The listing builds one solid part. Answer for the finished solid, in the listing's coordinates (mm). Face numbers are marked on the shaded views. Round coordinates to 2 decimals unless told otherwise and drop trailing zeros. Loops run counter-clockwise (first coordinate to the right, second up) from the corner with the lowest first, then second, coordinate; pieces in that order, holes last. Notation, with made-up numbers: (-15.5, -36.5) - (6.5, -36.5) arc R23 ccw to (6.5, -5.5) - close; hole circle Ø8 at (-39.75, 3). An arc over 180 degrees is marked (long way). Write item = value, one per line. Start each with the question number.
1) Section B-B, the plane x = 519 is taken. Determine the outline of the cut face in (y, z).
2) Section C-C, the plane y = 316.5 is taken. Determine the outline of the cut face in (x, z), and give its area (3 significant figures).
3) For a pull along Z with two mould halves and no side action, classify the marked faces 1 and 2 as released by +Z, released by -Z, zero draft, split by the parting line, or undercut.
4) Section A-A, the plane z = 0.45 is taken. Give the number of separate pieces and of enclosed holes in the cut face, and give its area (3 significant figures).
5) Given pin 1 Ø1.3 at (x, z) = (446.5, 1.5) entering from +Y; pin 2 Ø1 at (y, z) = (461.5, 1.5) entering from -X; pin 3 Ø0.5 at (x, z) = (446, 2) entering from -Y, each flat-ended and moving along its own axis, determine where each tip first touches the part or whether it passes through.
6) Straight lines are drawn through the part: line 1 along Y through (x, z) = (457, 2.9); line 2 along Y through (x, z) = (452.5, 0.1); line 3 along X through (y, z) = (567, 2.35). For each, find the intervals that lie inside material, in ascending order.
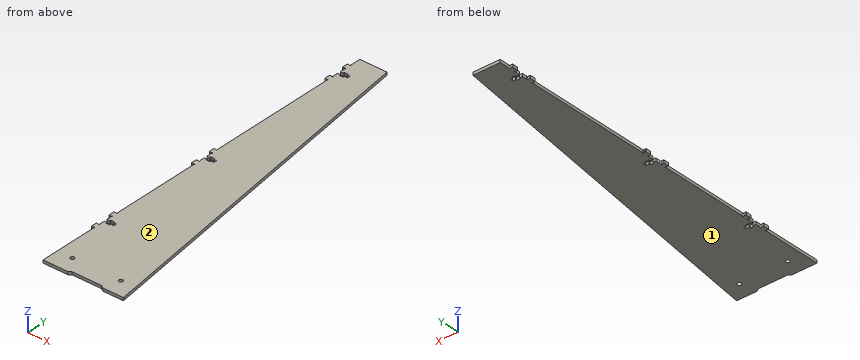
from build123d import *

# Parameters (mm, degrees)
MODEL_R                 = 2.05
SALIENTE_EXTRUIR1_DEPTH = 3


with BuildPart() as part:
    # Model → Saliente-Extruir1 (new body)
    with BuildSketch(Plane.XY):
        with BuildLine():
            Line((458.658091322, 643.996335498), (476.091013084, 643.996335498))
            Line((476.091013084, 643.996335498), (524.497055169, 308.953007972))
            Line((524.497055169, 308.953007972), (530.703308605, 265.996308498))
            Line((530.703308605, 265.996308498), (530.703308605, 263.996308498))
            Line((530.703308605, 263.996308498), (509.328287285, 263.996308498))
            Line((509.328287285, 263.996308498), (507.328283285, 265.996308498))
            Line((507.328283285, 265.996308498), (476.008092322, 265.996308498))
            Line((476.008092322, 265.996308498), (474.008092322, 263.996308498))
            Line((474.008092322, 263.996308498), (448.008092322, 263.996308498))
            Line((448.008092322, 263.996308498), (448.008095322, 324.530272498))
            ThreePointArc((448.008095322, 324.530272498), (448.075082188, 324.78027175), (448.258093826, 324.963284336))
            ThreePointArc((448.258093826, 324.963284336), (448.361645507, 325.749850684), (447.57507962, 325.646295498))
            ThreePointArc((447.57507962, 325.646295498), (447.39206666, 325.463282647), (447.142066322, 325.396295498))
            Line((447.142066322, 325.396295498), (445.508040322, 325.396292498))
            ThreePointArc((445.508040322, 325.396292498), (445.154486932, 325.542739108), (445.008040322, 325.896292498))
            Line((445.008040322, 325.896292498), (445.008040322, 330.896290498))
            ThreePointArc((445.008040322, 330.896290498), (445.154486932, 331.249843889), (445.508040322, 331.396290498))
            Line((445.508040322, 331.396290498), (447.142068322, 331.396290498))
            ThreePointArc((447.142068322, 331.396290498), (447.392067574, 331.329303632), (447.57508016, 331.146291995))
            ThreePointArc((447.57508016, 331.146291995), (448.361645749, 331.042740921), (448.258092322, 331.8293062))
            ThreePointArc((448.258092322, 331.8293062), (448.075079721, 332.012318727), (448.008092322, 332.262318498))
            Line((448.008092322, 332.262318498), (448.008092322, 337.396312498))
            Line((448.008092322, 337.396312498), (451.008064322, 337.396312498))
            Line((451.008064322, 337.396312498), (451.008064322, 336.121317498))
            Line((451.008064322, 336.121317498), (455.008092322, 336.121317498))
            Line((455.008092322, 336.121317498), (455.008092322, 337.396312498))
            Line((455.008092322, 337.396312498), (458.008092322, 337.396312498))
            Line((458.008092322, 337.396312498), (458.008092322, 340.596323498))
            Line((458.008092322, 340.596323498), (455.008092322, 340.596323498))
            Line((455.008092322, 340.596323498), (455.008092322, 341.871317498))
            Line((455.008092322, 341.871317498), (451.008064322, 341.871317498))
            Line((451.008064322, 341.871317498), (451.008064322, 340.596323498))
            Line((451.008064322, 340.596323498), (448.008092322, 340.596323498))
            Line((448.008092322, 340.596323498), (448.008095322, 345.730288498))
            ThreePointArc((448.008095322, 345.730288498), (448.075082188, 345.98028775), (448.258093826, 346.163300336))
            ThreePointArc((448.258093826, 346.163300336), (448.3616449, 346.949865925), (447.57507962, 346.846312498))
            ThreePointArc((447.57507962, 346.846312498), (447.39206666, 346.663299647), (447.142066322, 346.596312498))
            Line((447.142066322, 346.596312498), (445.508040322, 346.596309498))
            ThreePointArc((445.508040322, 346.596309498), (445.154486932, 346.742756108), (445.008040322, 347.096309498))
            Line((445.008040322, 347.096309498), (445.008040322, 352.096306498))
            ThreePointArc((445.008040322, 352.096306498), (445.154486932, 352.449859889), (445.508040322, 352.596306498))
            Line((445.508040322, 352.596306498), (447.142068322, 352.596306498))
            ThreePointArc((447.142068322, 352.596306498), (447.392067574, 352.529319632), (447.57508016, 352.346307995))
            ThreePointArc((447.57508016, 352.346307995), (448.361645749, 352.242756921), (448.258092322, 353.0293222))
            ThreePointArc((448.258092322, 353.0293222), (448.075079721, 353.212334727), (448.008092322, 353.462334498))
            Line((448.008092322, 353.462334498), (448.008095322, 353.464066546))
            Line((448.008095322, 353.464066546), (448.008095322, 444.530276498))
            ThreePointArc((448.008095322, 444.530276498), (448.075082188, 444.78027575), (448.258093826, 444.963288336))
            ThreePointArc((448.258093826, 444.963288336), (448.361645507, 445.749854684), (447.57507962, 445.646299498))
            ThreePointArc((447.57507962, 445.646299498), (447.39206666, 445.463286647), (447.142066322, 445.396299498))
            Line((447.142066322, 445.396299498), (445.508040322, 445.396296498))
            ThreePointArc((445.508040322, 445.396296498), (445.154486932, 445.542743108), (445.008040322, 445.896296498))
            Line((445.008040322, 445.896296498), (445.008040322, 450.896294498))
            ThreePointArc((445.008040322, 450.896294498), (445.154486932, 451.249847889), (445.508040322, 451.396294498))
            Line((445.508040322, 451.396294498), (447.142068322, 451.396294498))
            ThreePointArc((447.142068322, 451.396294498), (447.392067574, 451.329307632), (447.57508016, 451.146295995))
            ThreePointArc((447.57508016, 451.146295995), (448.361645749, 451.042744921), (448.258092322, 451.8293102))
            ThreePointArc((448.258092322, 451.8293102), (448.075079721, 452.012322727), (448.008092322, 452.262322498))
            Line((448.008092322, 452.262322498), (448.008092322, 457.396316498))
            Line((448.008092322, 457.396316498), (451.008064322, 457.396316498))
            Line((451.008064322, 457.396316498), (451.008064322, 456.121321498))
            Line((451.008064322, 456.121321498), (455.008092322, 456.121321498))
            Line((455.008092322, 456.121321498), (455.008092322, 457.396316498))
            Line((455.008092322, 457.396316498), (458.008092322, 457.396316498))
            Line((458.008092322, 457.396316498), (458.008092322, 460.596327498))
            Line((458.008092322, 460.596327498), (455.008092322, 460.596327498))
            Line((455.008092322, 460.596327498), (455.008092322, 461.871321498))
            Line((455.008092322, 461.871321498), (451.008064322, 461.871321498))
            Line((451.008064322, 461.871321498), (451.008064322, 460.596327498))
            Line((451.008064322, 460.596327498), (448.008092322, 460.596327498))
            Line((448.008092322, 460.596327498), (448.008095322, 465.730292498))
            ThreePointArc((448.008095322, 465.730292498), (448.075082188, 465.98029175), (448.258093826, 466.163304336))
            ThreePointArc((448.258093826, 466.163304336), (448.361645507, 466.949870684), (447.57507962, 466.846315498))
            ThreePointArc((447.57507962, 466.846315498), (447.39206666, 466.663302647), (447.142066322, 466.596315498))
            Line((447.142066322, 466.596315498), (445.508040322, 466.596312498))
            ThreePointArc((445.508040322, 466.596312498), (445.154486932, 466.742759108), (445.008040322, 467.096312498))
            Line((445.008040322, 467.096312498), (445.008040322, 472.096310498))
            ThreePointArc((445.008040322, 472.096310498), (445.154486932, 472.449863889), (445.508040322, 472.596310498))
            Line((445.508040322, 472.596310498), (447.142068322, 472.596310498))
            ThreePointArc((447.142068322, 472.596310498), (447.392067574, 472.529323632), (447.57508016, 472.346311995))
            ThreePointArc((447.57508016, 472.346311995), (448.361645749, 472.242760921), (448.258092322, 473.0293262))
            ThreePointArc((448.258092322, 473.0293262), (448.075081422, 473.212339245), (448.008095322, 473.462338498))
            Line((448.008095322, 473.462338498), (448.008095322, 473.464070546))
            Line((448.008095322, 473.464070546), (448.008095322, 604.530272498))
            ThreePointArc((448.008095322, 604.530272498), (448.075082188, 604.78027175), (448.258093826, 604.963284336))
            ThreePointArc((448.258093826, 604.963284336), (448.3616449, 605.749849925), (447.57507962, 605.646296498))
            ThreePointArc((447.57507962, 605.646296498), (447.39206666, 605.463283647), (447.142066322, 605.396296498))
            Line((447.142066322, 605.396296498), (445.508040322, 605.396293498))
            ThreePointArc((445.508040322, 605.396293498), (445.154486932, 605.542740108), (445.008040322, 605.896293498))
            Line((445.008040322, 605.896293498), (445.008040322, 610.896290498))
            ThreePointArc((445.008040322, 610.896290498), (445.154486932, 611.249843889), (445.508040322, 611.396290498))
            Line((445.508040322, 611.396290498), (447.142068322, 611.396290498))
            ThreePointArc((447.142068322, 611.396290498), (447.392067574, 611.329303632), (447.57508016, 611.146291995))
            ThreePointArc((447.57508016, 611.146291995), (448.361645749, 611.042740921), (448.258092322, 611.8293062))
            ThreePointArc((448.258092322, 611.8293062), (448.075079721, 612.012318727), (448.008092322, 612.262318498))
            Line((448.008092322, 612.262318498), (448.008092322, 617.396312498))
            Line((448.008092322, 617.396312498), (451.008064322, 617.396312498))
            Line((451.008064322, 617.396312498), (451.008064322, 616.121318498))
            Line((451.008064322, 616.121318498), (455.008092322, 616.121318498))
            Line((455.008092322, 616.121318498), (455.008092322, 617.396312498))
            Line((455.008092322, 617.396312498), (458.008092322, 617.396312498))
            Line((458.008092322, 617.396312498), (458.008092322, 620.596323498))
            Line((458.008092322, 620.596323498), (455.008092322, 620.596323498))
            Line((455.008092322, 620.596323498), (455.008092322, 621.871318498))
            Line((455.008092322, 621.871318498), (451.008064322, 621.871318498))
            Line((451.008064322, 621.871318498), (451.008064322, 620.596323498))
            Line((451.008064322, 620.596323498), (448.008092322, 620.596323498))
            Line((448.008092322, 620.596323498), (448.008095322, 625.730288498))
            ThreePointArc((448.008095322, 625.730288498), (448.075082188, 625.98028775), (448.258093826, 626.163300336))
            ThreePointArc((448.258093826, 626.163300336), (448.3616449, 626.949865925), (447.57507962, 626.846312498))
            ThreePointArc((447.57507962, 626.846312498), (447.39206666, 626.663299647), (447.142066322, 626.596312498))
            Line((447.142066322, 626.596312498), (445.508040322, 626.596309498))
            ThreePointArc((445.508040322, 626.596309498), (445.154486932, 626.742756108), (445.008040322, 627.096309498))
            Line((445.008040322, 627.096309498), (445.008040322, 632.096306498))
            ThreePointArc((445.008040322, 632.096306498), (445.154486932, 632.449859889), (445.508040322, 632.596306498))
            Line((445.508040322, 632.596306498), (447.142068322, 632.596306498))
            ThreePointArc((447.142068322, 632.596306498), (447.392067574, 632.529319632), (447.57508016, 632.346307995))
            ThreePointArc((447.57508016, 632.346307995), (448.361645749, 632.242756921), (448.258092322, 633.0293222))
            ThreePointArc((448.258092322, 633.0293222), (448.075079471, 633.21233516), (448.008092322, 633.462335498))
            Line((448.008092322, 633.462335498), (448.008092322, 643.996335498))
            Line((448.008092322, 643.996335498), (458.658091322, 643.996335498))
        make_face()
        with Locations((463.687972981, 280.996308498)):
            Circle(MODEL_R, mode=Mode.SUBTRACT)
        with Locations((513.687972981, 280.996308498)):
            Circle(MODEL_R, mode=Mode.SUBTRACT)
    extrude(amount=SALIENTE_EXTRUIR1_DEPTH)


solid = part.part
Geometry check:
q1.outline = (264, 0) - (347, 0) - (347, 3) - (264, 3) - close
q2.outline = (448.01, 0) - (523.41, 0) - (523.41, 3) - (448.01, 3) - close
q2.area = 226 mm2
q3.face_1 = released by -Z
q3.face_2 = released by +Z
q4.separate_pieces = 1
q4.enclosed_holes = 2
q4.area = 21,000 mm2
q5.pin_1 = 632.6
q5.pin_2 = 448.01
q5.pin_3 = 325.4
q6.line_1 = 264 to 337.4, 340.6 to 457.4, 460.6 to 617.4, 620.6 to 644
q6.line_2 = 264 to 336.12, 341.87 to 456.12, 461.87 to 616.12, 621.87 to 644
q6.line_3 = 448.01 to 487.22
